from build123d import *

# Parameters (mm, degrees)
BOSS_EXTRUDE1_DEPTH = 42
FILLET3_R           = 15
FILLET4_R           = 10
SHELL1_T            = -3
BOSS_EXTRUDE2_DEPTH = 39
CUT_EXTRUDE1_REACH  = 77.357
SKETCH4_W           = 10.2
SKETCH4_H           = 10.2
CUT_EXTRUDE2_DEPTH  = 10


with BuildPart() as part:
    # Sketch1 → Boss-Extrude1 (new body)
    with BuildSketch(Plane(origin=(0, 0, 0), x_dir=(1, 0, 0), z_dir=(0, 1, 0))):
        with BuildLine():
            Line((17.5, 0), (-17.5, 0))
            Line((-17.5, 0), (-38, 30))
            Line((-38, 30), (-38, 40))
            ThreePointArc((-38, 40), (0, 50), (38, 40))
            Line((38, 40), (38, 30))
            Line((38, 30), (17.5, 0))
        make_face()
    extrude(amount=BOSS_EXTRUDE1_DEPTH)

    # Fillet3
    fillet3_edges = [part.edges().sort_by_distance(p)[0] for p in [
        (-38, 21, -40),
        (38, 21, -40),
    ]]
    fillet(fillet3_edges, radius=FILLET3_R)

    # Fillet4
    fillet4_edges = [part.edges().sort_by_distance(p)[0] for p in [
        (38, 21, -30),
        (-38, 21, -30),
    ]]
    fillet(fillet4_edges, radius=FILLET4_R)

    # Shell1
    shell1_openings = [part.faces().sort_by_distance(p)[0] for p in [
        (0, 42, -26.142046548),
    ]]
    offset(amount=SHELL1_T, openings=shell1_openings)

    # Sketch3 → Boss-Extrude2 (add)
    with BuildSketch(Plane(origin=(0, 42, 0), x_dir=(1, 0, 0), z_dir=(0, 1, 0))):
        Polygon((-20.699808874, 10), (20.699808874, 10), (15.91647554, 3), (-15.91647554, 3), align=None)
    extrude(amount=-BOSS_EXTRUDE2_DEPTH)

    # Sketch4 → Cut-Extrude1 (cut, up to next)
    with BuildSketch(Plane.XY, mode=Mode.PRIVATE) as cut_extrude1_sk1:
        with Locations((0, 24)):
            Rectangle(SKETCH4_W, SKETCH4_H)
    cut_extrude1_tool1 = extrude(cut_extrude1_sk1.sketch, amount=-CUT_EXTRUDE1_REACH, mode=Mode.PRIVATE) & part.part
    add(cut_extrude1_tool1.solids().sort_by_distance((0, 24, 0))[0], mode=Mode.SUBTRACT)

    # Sketch5 → Cut-Extrude2 (cut)
    with BuildSketch(Plane(origin=(0, 42, 0), x_dir=(1, 0, 0), z_dir=(0, 1, 0))):
        with BuildLine():
            Line((-10, 10), (10, 10))
            ThreePointArc((10, 10), (0, 3.582575695), (-10, 10))
        make_face()
    extrude(amount=-CUT_EXTRUDE2_DEPTH, mode=Mode.SUBTRACT)


solid = part.part
Source: CAD feature listing. Evaluate the final solid. Frame: model axes, mm. A direction names the side the tool comes from. Round coordinates to 2 decimals unless told otherwise and drop trailing zeros. Loops run counter-clockwise (first coordinate to the right, second up) from the corner with the lowest first, then second, coordinate; pieces in that order, holes last. Notation, with made-up numbers: M -24,32 L 30,32 A22 cw 30,60 Z; hole C -9,81.25 d4. An arc over 180 degrees is marked long. Return JSON: item names as keys, results as strings. Group by question number.
1. Pin query (flat end, axial travel): pin 1 (5 mm diameter, centred on y = 22, z = -3.5, fed in from +X); pin 2 (18.5 mm diameter, centred on x = 1, z = -26.5, fed in from +Y); pin 3 (4 mm diameter, centred on y = 9.5, z = -18, fed in from -X). Return the tip coordinate at first contact, or that it passes through.
2. Section query C-C on x = 18.5. Output: boundary loops of the cut face in (y, z).
3. Section query D-D on z = -23.5. Output: boundary loops of the cut face in (x, y).
4. Section query A-A on x = -4. Output: boundary loops of the cut face in (y, z), and give its area (3 significant figures).
5. Reachability of faces 1 (the face through (0, 18.9, -5)), 2 (the face through (0, 32, -8)), 3 (the face through (-26.556, 20.706, -13.252)) from +Z, -Z, +X, -X, +Y, -Y: full face, straight path, thin tool, end or side. Return the list, or none.
6. Section query B-B on z = -8. Output: boundary loops of the cut face in (x, y), and give its area (3 significant figures).
7. Material intervals for line 1 along X through (y, z) = (20, -32); line 2 along Y through (x, z) = (0.5, -3); line 3 along Y through (x, z) = (12, -39), sorted ascending. Write a range as from..to.
8. Mould query, pull axis Y, two halves, no side actions, for faces 4 (the face through (-8.2, 42, -6.6)), 5 (the face through (0, 16, 0)), 6 (the face through (-5.1, 24, -5)). Classes: released by +Y, released by -Y, zero draft, split by the parting line, or undercut.
Checks:
{
 "1": {"pin 1": "stops at x = 21.6", "pin 2": "stops at y = 3", "pin 3": "stops at x = -31.17"},
 "2": {"outline": "M 0,-47.75 L 42,-47.75 L 42,-44.66 L 3,-44.66 L 3,-10 L 42,-10 L 42,-1.46 L 0,-1.46 Z"},
 "3": {"outline": "M -33.56,0 L 33.56,0 L 33.56,42 L 29.92,42 L 29.92,3 L -29.92,3 L -29.92,42 L -33.56,42 Z"},
 "4": {"outline": "M 0,-49.9 L 42,-49.9 L 42,-46.89 L 3,-46.89 L 3,-10 L 18.9,-10 L 18.9,0 L 0,0 Z; M 29.1,-10 L 32,-10 L 32,-4.34 L 42,-4.34 L 42,0 L 29.1,0 Z", "area": "498 mm²"},
 "5": {"face 1": "+Z", "face 2": "+Y", "face 3": "+Z, -X, +Y, -Y"},
 "6": {"outline": "M -22.97,0 L 22.97,0 L 22.97,42 L 8.81,42 L 8.81,32 L -8.81,32 L -8.81,42 L -22.97,42 Z; hole M -5.1,18.9 L 5.1,18.9 L 5.1,29.1 L -5.1,29.1 Z", "area": "1,650 mm²"},
 "7": {"line 1": "x = -37.6..-34.59, 34.59..37.6", "line 2": "y = 0..18.9, 29.1..42", "line 3": "y = 0..3"},
 "8": {"face 4": "released by +Y", "face 5": "zero draft", "face 6": "undercut"}
}
